Here's how the part is built. I have some questions about the finished solid (model axes, mm). Face numbers are marked on the shaded views. Coordinates: 2 decimals unless noted, no trailing zeros. Write each loop counter-clockwise with the first axis right and the second up, starting at its lowest first coordinate (ties: lowest second). Pieces come first, ordered by that corner, then holes. Notation, with made-up numbers: (0, 76.25) -> (14, 76.25) arc R6 cw to (14, 83.25) -> close; hole circle Ø6 at (19, 8). An arc over 180 degrees is marked (long way). Put each result on its own line as item: value. Start each with the question number.
Item 1: I want a section at C-C, the plane z = 14. List the corners of the cut face in (x, y) for me.
Item 2: For pin 1 (6 mm diameter, centred on x = 50.29, y = -29.04, fed in from +Z); pin 2 (3 mm diameter, centred on x = -44.54, y = -25.72, fed in from +Z); pin 3 (6 mm diameter, centred on x = -50, y = -30.5, fed in from +Z); pin 4 (6 mm diameter, centred on y = 34.5, z = 13.5, fed in from -X), each with a flat end and sliding along its axis, tell me the tip position at first contact or that it passes through.
Item 3: If we mould it in two halves opening along X, with no side actions, what happens to the marked faces 1, 2 and 3? For each: released by +X, released by -X, zero draft, split by the parting line, or undercut.
Item 4: I need wall thicknesses on line 1 (X direction, y = -5.5, z = 2); line 2 (X direction, y = 1, z = 9.5); line 3 (Z direction, x = -25.5, y = 14.5). Which ranges of each line are inside material? Lowest first, please. Write a range as [from, to].
Item 5: I want a section at D-D, the plane x = 0. State how many separate pieces and enclosed holes the cut face has, then the cut area to 3 significant figures.
Item 6: I want a section at A-A, the plane y = 0. List the corners of the cut face in (x, z) for me, then the cut area to 3 significant figures.
Item 7: I want a section at B-B, the plane x = 20. List the corners of the cut face in (y, z) for me.
from build123d import *

# Parameters (mm, degrees)
SKETCH1_R                    = 66.8
SKETCH1_R_2                  = 63.5
BOSS_EXTRUDE1_DEPTH          = 15.88
SKETCH2_R                    = 63.5
BOSS_EXTRUDE2_DEPTH          = 3.18
CUT_EXTRUDE2_DEPTH           = 96.319305495
SKETCH5_R                    = 4.7625
SKETCH5_R_2                  = 3.18
CUT_EXTRUDE1_DEPTH           = 96.319305495
CIRPATTERN2_COUNT            = 3
CIRPATTERN3_COUNT            = 2
HOLE1_D                      = 3.2639
CIRPATTERN5_COUNT            = 3
CIRPATTERN5_ANGLE            = 240
HOLE2_D                      = 3.2639
CIRPATTERN6_COUNT            = 3
F_1_0_1_DIAMETER_HOLE1_D     = 7.239
F_1_0_1_DIAMETER_HOLE1_DEPTH = 1.1176
CIRPATTERN7_COUNT            = 3


with BuildPart() as part:
    # Sketch1 → Boss-Extrude1 (new body)
    with BuildSketch(Plane.XY):
        Circle(SKETCH1_R)
        Circle(SKETCH1_R_2, mode=Mode.SUBTRACT)
    extrude(amount=BOSS_EXTRUDE1_DEPTH)

    # Sketch2 → Boss-Extrude2 (add)
    with BuildSketch(Plane.XY):
        Circle(SKETCH2_R)
    extrude(amount=BOSS_EXTRUDE2_DEPTH)

    # Sketch6 → Cut-Extrude2 (cut, through all)
    with BuildSketch(Plane.XY.offset(3.18)):
        with BuildLine():
            ThreePointArc((-23.927369503, 50.442160591), (-48.348915265, 27.916177552), (-55.64814492, -4.496058651))
            ThreePointArc((-55.64814492, -4.496058651), (-54.328981929, -8.966343359), (-51.327740035, -12.532319168))
            ThreePointArc((-51.327740035, -12.532319168), (-37.384150369, -14.226795935), (-30.412116254, -2.033121978))
            ThreePointArc((-30.412116254, -2.033121978), (-26.421749263, 15.196103641), (-13.536182991, 27.309378426))
            ThreePointArc((-13.536182991, 27.309378426), (-6.368971607, 39.443915619), (-14.817446368, 50.723950466))
            ThreePointArc((-14.817446368, 50.723950466), (-19.40184977, 51.534874128), (-23.927369503, 50.442160591))
        make_face()
    cut_extrude2 = extrude(amount=-CUT_EXTRUDE2_DEPTH, mode=Mode.SUBTRACT)

    # Sketch5 → Cut-Extrude1 (cut, through all)
    with BuildSketch(Plane.XY.offset(3.18)):
        Circle(SKETCH5_R)
        with Locations((0, 19.05)):
            Circle(SKETCH5_R_2)
    cut_extrude1 = extrude(amount=-CUT_EXTRUDE1_DEPTH, mode=Mode.SUBTRACT)

    # CirPattern2: Cut-Extrude2 ×3 about axis
    cirpattern2_axis = Axis((0, 0, 0), (0, 0, 1))
    for i in range(1, CIRPATTERN2_COUNT):
        add(cut_extrude2.rotate(cirpattern2_axis, i * 360 / CIRPATTERN2_COUNT), mode=Mode.SUBTRACT)

    # CirPattern3: Cut-Extrude1 ×2 about axis
    cirpattern3_axis = Axis((0, 0, 0), (0, 0, 1))
    for i in range(1, CIRPATTERN3_COUNT):
        add(cut_extrude1.rotate(cirpattern3_axis, i * 360 / CIRPATTERN3_COUNT), mode=Mode.SUBTRACT)

    # Hole1 (through all)
    with Locations(Plane(origin=(0, 0, 0), x_dir=(-1, 0, 0), z_dir=(0, 0, -1))):
        with Locations((0, 58.07456)):
            hole1 = Hole(HOLE1_D / 2)

    # CirPattern5: Hole1 ×3 about axis
    cirpattern5_axis = Axis((0, 0, 0), (0, 0, 1))
    for i in range(1, CIRPATTERN5_COUNT):
        add(hole1.rotate(cirpattern5_axis, i * CIRPATTERN5_ANGLE / (CIRPATTERN5_COUNT - 1)), mode=Mode.SUBTRACT)

    # Hole2 (through all)
    with Locations(Plane(origin=(0, 0, 0), x_dir=(-1, 0, 0), z_dir=(0, 0, -1))):
        with Locations((0, 51.435)):
            hole2 = Hole(HOLE2_D / 2)

    # CirPattern6: Hole2 ×3 about axis
    cirpattern6_axis = Axis((0, 0, 0), (0, 0, 1))
    for i in range(1, CIRPATTERN6_COUNT):
        add(hole2.rotate(cirpattern6_axis, i * 360 / CIRPATTERN6_COUNT), mode=Mode.SUBTRACT)

    # Ø1.0 (1) Diameter Hole1
    with Locations(Plane(origin=(0, 58.07456, 3.18), x_dir=(1, 0, 0), z_dir=(0, 0, 1))):
        with Locations((0, 0)):
            f_1_0_1_diameter_hole1 = Hole(F_1_0_1_DIAMETER_HOLE1_D / 2, depth=F_1_0_1_DIAMETER_HOLE1_DEPTH)

    # CirPattern7: Ø1.0 (1) Diameter Hole1 ×3 about axis
    cirpattern7_axis = Axis((0, 0, 0), (0, 0, 1))
    for i in range(1, CIRPATTERN7_COUNT):
        add(f_1_0_1_diameter_hole1.rotate(cirpattern7_axis, i * 360 / CIRPATTERN7_COUNT), mode=Mode.SUBTRACT)


solid = part.part
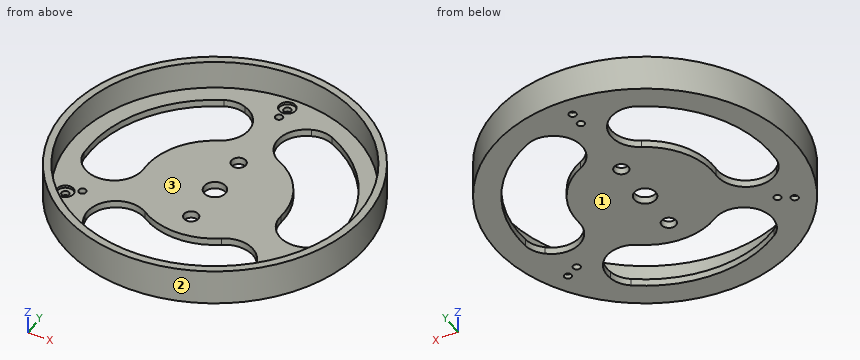
Calculated:
1. outline: circle Ø133.6 at (0, 0); hole circle Ø127 at (0, 0)
2. pin 1: stops at z = 2.06
2. pin 2: passes through
2. pin 3: stops at z = 3.18
2. pin 4: stops at x = -58.91
3. face 1: zero draft
3. face 2: split by the parting line
3. face 3: undercut
4. line 1: x = [-66.57, -55.52], [-30.66, 30.66], [55.52, 66.57]
4. line 2: x = [-66.79, -63.49], [63.49, 66.79]
4. line 3: z = [0, 3.18]
5. separate pieces: 7
5. enclosed holes: 0
5. area: 332 mm2
6. outline: (-66.8, 0) -> (-55.83, 0) -> (-55.83, 3.18) -> (-63.5, 3.18) -> (-63.5, 15.88) -> (-66.8, 15.88) -> close; (-30.48, 0) -> (-4.76, 0) -> (-4.76, 3.18) -> (-30.48, 3.18) -> close; (4.76, 0) -> (30.48, 0) -> (30.48, 3.18) -> (4.76, 3.18) -> close; (55.83, 0) -> (66.8, 0) -> (66.8, 15.88) -> (63.5, 15.88) -> (63.5, 3.18) -> (55.83, 3.18) -> close
6. area: 317 mm2
7. outline: (-63.74, 0) -> (-52.12, 0) -> (-52.12, 3.18) -> (-60.27, 3.18) -> (-60.27, 15.88) -> (-63.74, 15.88) -> close; (-23.83, 0) -> (23, 0) -> (23, 3.18) -> (-23.83, 3.18) -> close; (51.5, 0) -> (63.74, 0) -> (63.74, 15.88) -> (60.27, 15.88) -> (60.27, 3.18) -> (51.5, 3.18) -> close
